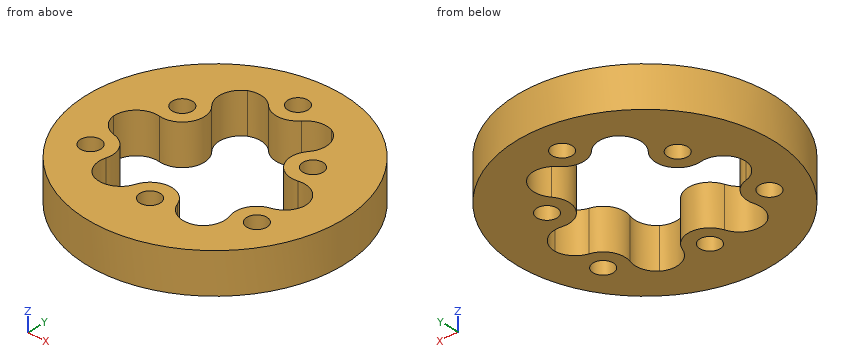
```python
from build123d import *

# Parameters (mm, degrees)
ESQUISSE1_R        = 19
ESQUISSE1_R_2      = 1.5
BOSS_EXTRU_2_DEPTH = 6


with BuildPart() as part:
    # Esquisse1 → Boss.-Extru.2 (new body)
    with BuildSketch(Plane.XY):
        Circle(ESQUISSE1_R)
        with Locations((-0.493805045, 13.991288596)):
            Circle(ESQUISSE1_R_2, mode=Mode.SUBTRACT)
        with Locations((12.363713879, -6.567996584)):
            Circle(ESQUISSE1_R_2, mode=Mode.SUBTRACT)
        with Locations((-11.869908833, -7.423292012)):
            Circle(ESQUISSE1_R_2, mode=Mode.SUBTRACT)
        with Locations((-9.714346619, 5.160568745)):
            Circle(ESQUISSE1_R_2, mode=Mode.SUBTRACT)
        with Locations((9.32635694, 5.832586581)):
            Circle(ESQUISSE1_R_2, mode=Mode.SUBTRACT)
        with Locations((0.387989679, -10.993155325)):
            Circle(ESQUISSE1_R_2, mode=Mode.SUBTRACT)
        with BuildLine():
            ThreePointArc((-2.815595301, 11.717131607), (-0.379171731, 10.743310886), (1.982535482, 11.886475637))
            ThreePointArc((1.982535482, 11.886475637), (3.675716254, 12.935891711), (5.663115611, 12.800322476))
            ThreePointArc((5.663115611, 12.800322476), (7.409047573, 10.596596907), (6.782830345, 7.855696182))
            ThreePointArc((6.782830345, 7.855696182), (6.57084239, 4.109322364), (10.032070946, 2.660132051))
            ThreePointArc((10.032070946, 2.660132051), (12.770566856, 2.023480694), (13.987784639, -0.510896087))
            ThreePointArc((13.987784639, -0.510896087), (13.239790253, -2.357146239), (11.555131282, -3.420188746))
            ThreePointArc((11.555131282, -3.420188746), (9.493566014, -5.043283091), (9.302722122, -7.66016391))
            ThreePointArc((9.302722122, -7.66016391), (9.364952716, -9.651209509), (8.253846635, -11.304563222))
            ThreePointArc((8.253846635, -11.304563222), (5.472398329, -11.71472187), (3.411817286, -9.80195148))
            ThreePointArc((3.411817286, -9.80195148), (0.273356364, -7.745177616), (-2.712293539, -10.018094318))
            ThreePointArc((-2.712293539, -10.018094318), (-4.632897743, -12.071375665), (-7.436341309, -11.858328797))
            ThreePointArc((-7.436341309, -11.858328797), (-8.66124365, -10.287421581), (-8.739535981, -8.296942861))
            ThreePointArc((-8.739535981, -8.296942861), (-9.114394283, -5.700027795), (-11.285257604, -4.226311727))
            ThreePointArc((-11.285257604, -4.226311727), (-13.04066897, -3.284682203), (-13.916962247, -1.495759254))
            ThreePointArc((-13.916962247, -1.495759254), (-12.881445902, 1.118124963), (-10.194647631, 1.946255297))
            ThreePointArc((-10.194647631, 1.946255297), (-6.844198754, 3.635855252), (-7.319777407, 7.357962266))
            ThreePointArc((-7.319777407, 7.357962266), (-8.137669113, 10.047894971), (-6.55144333, 12.369224883))
            ThreePointArc((-6.55144333, 12.369224883), (-4.578546604, 12.64456782), (-2.815595301, 11.717131607))
        make_face(mode=Mode.SUBTRACT)
    extrude(amount=BOSS_EXTRU_2_DEPTH)


solid = part.part
```
The listing builds one solid part. Answer for the finished solid, in the listing's coordinates (mm). Give positions to 0.01 mm unless a question says otherwise; leave off trailing zeros. Write each loop counter-clockwise with the first axis right and the second up, starting at its lowest first coordinate (ties: lowest second). Pieces come first, ordered by that corner, then holes. Notation, with made-up numbers: (-24, -32.5) - (0, -32.5) arc R10 ccw to (0, -13.5) - close; hole circle Ø1 at (-1, 75.5). An arc over 180 degrees is marked (long way). Use one line per item in the form item = value. Start each with the question number.
1) Flat-ended cylindrical pins translate along their axes: pin 1 Ø2 at (x, z) = (11, 3) entering from +Y; pin 2 Ø5 at (x, y) = (3, -4) entering from +Z; pin 3 Ø1.5 at (y, z) = (7, 3.5) entering from +X. Find the tip coordinate at first contact, or state that the pin passes through.
2) Find section C-C on z = 2.25. Determine the outline of the cut face in (x, y), plus the area to 3 significant figures.
3) Find section B-B on y = 10. Determine the outline of the cut face in (x, z).
4) Consider line 1 along Y through (x, z) = (8, 4.9); line 2 along Y through (x, z) = (-12, 3.25); line 3 along X through (y, z) = (4, 5.35). Determine where each line is inside the solid, lowest interval first. Write a range as from..to.
5) Find section D-D on x = -6. Determine the outline of the cut face in (y, z), plus the area to 3 significant figures.
6) Find section A-A on x = 0. Determine the outline of the cut face in (y, z), plus the area to 3 significant figures.
Geometry results:
q1.pin_1 = 16.16
q1.pin_2 = through
q1.pin_3 = 17.94
q2.outline = circle Ø38 at (0, 0); hole (-13.92, -1.5) arc R3.25 ccw to (-11.29, -4.23) arc R3.25 cw to (-8.74, -8.3) arc R3.25 ccw to (-7.44, -11.86) arc R3.25 ccw to (-2.71, -10.02) arc R3.25 cw to (3.41, -9.8) arc R3.25 ccw to (8.25, -11.3) arc R3.25 ccw to (9.3, -7.66) arc R3.25 cw to (11.56, -3.42) arc R3.25 ccw to (13.99, -0.51) arc R3.25 ccw to (10.03, 2.66) arc R3.25 cw to (6.78, 7.86) arc R3.25 ccw to (5.66, 12.8) arc R3.25 ccw to (1.98, 11.89) arc R3.25 cw to (-2.82, 11.72) arc R3.25 ccw to (-6.55, 12.37) arc R3.25 ccw to (-7.32, 7.36) arc R3.25 cw to (-10.19, 1.95) arc R3.25 ccw to start; hole circle Ø3 at (-11.87, -7.42); hole circle Ø3 at (-9.71, 5.16); hole circle Ø3 at (-0.49, 13.99); hole circle Ø3 at (0.39, -10.99); hole circle Ø3 at (9.33, 5.83); hole circle Ø3 at (12.36, -6.57)
q2.area = 667 mm2
q3.outline = (-16.16, 0) - (-8.14, 0) - (-8.14, 6) - (-16.16, 6) - close; (7.49, 0) - (16.16, 0) - (16.16, 6) - (7.49, 6) - close
q4.line_1 = -17.23..-11.46, 2.87..5.13, 6.53..17.23
q4.line_2 = -14.73..-8.92, -5.93..-4.01, 1.7..14.73
q4.line_3 = -18.57..-10.66, -8.76..-6.68, 6.64..18.57
q5.outline = (-18.03, 0) - (-12.29, 0) - (-12.29, 6) - (-18.03, 6) - close; (12.58, 0) - (18.03, 0) - (18.03, 6) - (12.58, 6) - close
q5.area = 67.1 mm2
q6.outline = (-19, 0) - (-12.44, 0) - (-12.44, 6) - (-19, 6) - close; (-9.54, 0) - (-7.77, 0) - (-7.77, 6) - (-9.54, 6) - close; (10.78, 0) - (12.57, 0) - (12.57, 6) - (10.78, 6) - close; (15.41, 0) - (19, 0) - (19, 6) - (15.41, 6) - close
q6.area = 82.3 mm2
